from build123d import *

# Parameters (mm, degrees)
PAD_DEPTH       = 15
SKETCH001_R     = 2.25
POCKET_DEPTH    = 35.001
SKETCH002_R     = 2.25
POCKET001_DEPTH = 45.001
SKETCH003_R     = 5
POCKET002_DEPTH = 36
SKETCH004_W     = 65
SKETCH004_H     = 10
PAD001_DEPTH    = 15
SKETCH005_R     = 2.019914
SKETCH005_R_2   = 14
POCKET003_DEPTH = 55.001
SKETCH006_R     = 4
POCKET004_DEPTH = 5
FILLET_R        = 3
FILLET001_R     = 4
FILLET002_R     = 2


with BuildPart() as part:
    # Sketch → Pad (new body)
    with BuildSketch(Plane.XY):
        with BuildLine():
            Line((45, 15), (-20, 15))
            Line((-20, 15), (-20, -20))
            Line((0, -20), (-20, -20))
            Line((0, -40), (0, -20))
            Line((0, -40), (10, -40))
            Line((10, -40), (10, -35.000001))
            ThreePointArc((45, 0), (20.251262, -10.251263), (10, -35.000001))
            Line((45, 0), (45, 15))
        make_face()
    extrude(amount=PAD_DEPTH)

    # Sketch001 → Pocket (cut, through all)
    with BuildSketch(Plane.XZ.offset(20)):
        with Locations((-10, 7.5)):
            Circle(SKETCH001_R)
    extrude(amount=-POCKET_DEPTH, mode=Mode.SUBTRACT)

    # Sketch002 → Pocket001 (cut, through all)
    with BuildSketch(Plane(origin=(0, 0, 0), x_dir=(0, -1, 0), z_dir=(-1, 0, 0))):
        with Locations((30, 7.5)):
            Circle(SKETCH002_R)
    extrude(amount=-POCKET001_DEPTH, mode=Mode.SUBTRACT)

    # Sketch003 → Pocket002 (cut)
    with BuildSketch(Plane.YZ.offset(45)):
        with Locations((-30, 7.5)):
            Circle(SKETCH003_R)
    extrude(amount=-POCKET002_DEPTH, mode=Mode.SUBTRACT)

    # Sketch004 → Pad001 (new body)
    with BuildSketch(Plane.XY.offset(15)):
        with Locations((12.5, 10)):
            Rectangle(SKETCH004_W, SKETCH004_H)
    extrude(amount=PAD001_DEPTH)

    # Sketch005 → Pocket003 (cut, through all)
    with BuildSketch(Plane(origin=(0, 15, 0), x_dir=(-1, 0, 0), z_dir=(0, 1, 0))):
        with Locations((-37.5, 24.5)):
            Circle(SKETCH005_R)
        with Locations((-6.5, 24.5)):
            Circle(SKETCH005_R)
        with Locations((-22, 40)):
            Circle(SKETCH005_R_2)
    extrude(amount=-POCKET003_DEPTH, mode=Mode.SUBTRACT)

    # Sketch006 → Pocket004 (cut)
    with BuildSketch(Plane(origin=(0, 15, 0), x_dir=(-1, 0, 0), z_dir=(0, 1, 0))):
        with Locations((-37.5, 24.5)):
            Circle(SKETCH006_R)
        with Locations((-6.5, 24.5)):
            Circle(SKETCH006_R)
    extrude(amount=-POCKET004_DEPTH, mode=Mode.SUBTRACT)

    # Fillet
    fillet_edges = [part.edges().sort_by_distance(p)[0] for p in [
        (12.5, 5, 15),
    ]]
    fillet(fillet_edges, radius=FILLET_R)

    # Fillet001
    fillet001_edges = [part.edges().sort_by_distance(p)[0] for p in [
        (-20, 10, 30),
        (45, 10, 30),
    ]]
    fillet(fillet001_edges, radius=FILLET001_R)

    # Fillet002
    fillet002_edges = [part.edges().sort_by_distance(p)[0] for p in [
        (45, 0, 7.5),
        (10, -40, 7.5),
    ]]
    fillet(fillet002_edges, radius=FILLET002_R)


solid = part.part
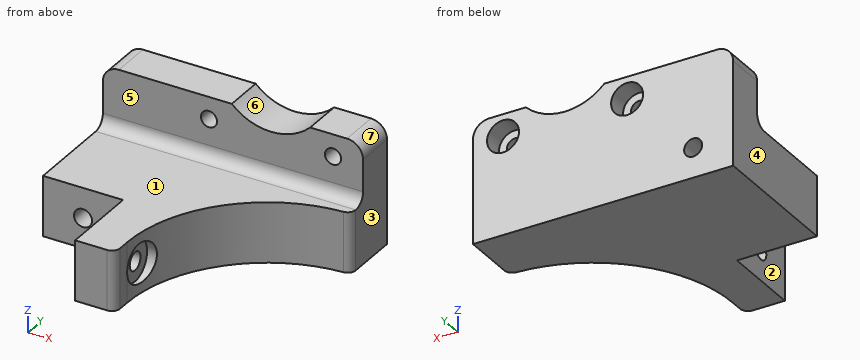
The model under review builds one solid part; all positions refer to its coordinate system, in mm. Face numbers are marked on the shaded views. A direction names the side the tool comes from. Give positions to 0.01 mm unless a question says otherwise; leave off trailing zeros. Loops run counter-clockwise (first coordinate to the right, second up) from the corner with the lowest first, then second, coordinate; pieces in that order, holes last. Notation, with made-up numbers: (6, -0.75) -> (29, -0.75) arc R20 cw to (29, 10.25) -> close; hole circle Ø7 at (-38, -22). An arc over 180 degrees is marked (long way). Put each result on its own line as item: value. Start each with the question number.
1. Mouldability with a two-part tool opening along X and no side actions: class the marked faces 4, 5, 6 and 7 as released by +X, released by -X, zero draft, split by the parting line, or undercut.
2. We need section D-D on y = -30. State the section outline as (x, z) points.
3. Clearance check with flat-ended pins moving along their axes: P1, Ø1.5, axis at y = -36.5, z = 10.5, coming from the +X side; P2, Ø4, axis at y = -25.5, z = 8.5, coming from the -X side; P3, Ø6, axis at x = 24, y = 1.5, coming from the +Z side; P4, Ø10.5, axis at x = 37.5, z = 24.5, coming from the +Y side. State where each tip first meets the part, or that it passes through.
4. Wall thickness on probe 1 along Z at (x, y) = (6.5, 7.85); probe 2 along Z at (x, y) = (2.25, -30); probe 3 along Y at (x, z) = (-11, 25): over which ranges is each line inside the solid? List them lowest first.
5. For the marked faces 1, 2 and 3, list the 3-axis set-ups (+Z, -Z, +X, -X, +Y, -Y) from which the entire face can be reached by the end or side of a thin tool; tool diameter is ignored.
6. We need section C-C on z = 9. State the section outline as (x, y) points, then the cut area to 3 significant figures.
7. We need section A-A on x = -10. State the section outline as (y, z) points, then the cut area to 3 significant figures.
8. We need section B-B on x = 6.5. State the section outline as (y, z) points, then the cut area to 3 significant figures.
Determined:
1. face 4: released by -X
1. face 5: zero draft
1. face 6: undercut
1. face 7: released by +X
2. outline: (0, 0) -> (10.36, 0) -> (10.36, 2.5) -> (9, 2.5) -> (9, 5.25) -> (0, 5.25) -> close; (0, 9.75) -> (9, 9.75) -> (9, 12.5) -> (10.36, 12.5) -> (10.36, 15) -> (0, 15) -> close
3. P1: x = 10
3. P2: x = 0
3. P3: z = 16.34
3. P4: y = 15
4. probe 1: 0 to 22.48, 26.52 to 30
4. probe 2: 0 to 5.25, 9.75 to 15
4. probe 3: 5 to 15
5. face 1: +Z, +X, -X, -Y
5. face 2: +Z, -Z, -X, -Y
5. face 3: +Z, -Z, +X, +Y, -Y
6. outline: (-20, -20) -> (-11.68, -20) -> (-11.68, 15) -> (-20, 15) -> close; (-8.32, -20) -> (0, -20) -> (0, -28.32) -> (9, -28.32) -> (9, -25.23) -> (11.39, -25.23) arc R35 cw to (43.11, -0.05) arc R2 ccw to (45, 1.95) -> (45, 15) -> (-8.32, 15) -> close; (0, -40) -> (8, -40) arc R2 ccw to (10, -38) -> (10, -35) arc R35 cw to (10, -34.77) -> (9, -34.77) -> (9, -31.68) -> (0, -31.68) -> close
6. area: 1,870 mm^2
7. outline: (-20, 0) -> (15, 0) -> (15, 5.25) -> (-20, 5.25) -> close; (-20, 9.75) -> (15, 9.75) -> (15, 30) -> (5, 30) -> (5, 18) arc R3 cw to (2, 15) -> (-20, 15) -> close
7. area: 519 mm^2
8. outline: (-40, 0) -> (15, 0) -> (15, 20.5) -> (10, 20.5) -> (10, 22.48) -> (5, 22.48) -> (5, 18) arc R3 cw to (2, 15) -> (-40, 15) -> close; (5, 26.52) -> (10, 26.52) -> (10, 28.5) -> (15, 28.5) -> (15, 30) -> (5, 30) -> close; hole circle Ø4.5 at (-30, 7.5)
8. area: 901 mm^2
